Work out the finished part from the listing and answer in its coordinate system (mm). A direction names the side the tool comes from. Coordinates: 2 decimals unless noted, no trailing zeros. Write each loop counter-clockwise with the first axis right and the second up, starting at its lowest first coordinate (ties: lowest second). Pieces come first, ordered by that corner, then holes. Notation, with made-up numbers: (7.5, 42) - (27.5, 42) arc R29 cw to (27.5, 63) - close; hole circle Ø5 at (16, 87.5). An arc over 180 degrees is marked (long way). Use one line per item in the form item = value. Start each with the question number.
Item 1: Given pin 1 (2 mm diameter, centred on x = 1855, z = -24.5, fed in from +Y), flat-ended and moving along its own axis, determine where the tip first touches the part or whether it passes through.
Item 2: A cutting plane is placed at C-C (x = 1818). Write down the section's boundary in (y, z) (3 decimals).
Item 3: For faces 1 (the cylindrical face through (1867, -21, 28)), 2 (the flat face through (1773.643, -0.499, -36.897)), determine the directions among +Z, -Z, +X, -X, +Y, -Y from which every point of the face is accessible in a straight line to the end or side of a thin tool.
Item 4: A cutting plane is placed at B-B (y = 12). Write down the section's boundary in (x, z) (3 decimals).
Item 5: Consider probe 1 along X at (y, z) = (26.5, 31); probe 2 along X at (y, z) = (-8, -14); probe 3 along Y at (x, z) = (1794, -25.5) (1 decimal). Determine where each line is inside the solid, lowest interval first.
Item 6: A cutting plane is placed at A-A (z = 0). Write down the section's boundary in (x, y) (3 decimals).
Item 7: A cutting plane is placed at D-D (y = 29.5). Write down the section's boundary in (x, z) (3 decimals).
from build123d import *

# Parameters (mm, degrees)
SKETCH1_W           = 76.33
SKETCH1_H           = 76.33
BOSS_EXTRUDE1_DEPTH = 76.33
SKETCH2_R           = 35
BOSS_EXTRUDE2_DEPTH = 36.82
CHAMFER1_SIZE       = 2.5
CUT_EXTRUDE1_REACH  = 78.33
SKETCH3_R           = 18.71


with BuildPart() as part:
    # Sketch1 → Boss-Extrude1 (new body)
    with BuildSketch(Plane.ZY.offset(-1848.740517551)):
        Rectangle(SKETCH1_W, SKETCH1_H)
    extrude(amount=BOSS_EXTRUDE1_DEPTH)

    # Sketch2 → Boss-Extrude2 (add)
    with BuildSketch(Plane(origin=(1848.740517551, 0, 0), x_dir=(0, 0, -1), z_dir=(1, 0, 0))):
        Circle(SKETCH2_R)
    extrude(amount=BOSS_EXTRUDE2_DEPTH)

    # Chamfer1
    chamfer1_edges = [part.edges().sort_by_distance(p)[0] for p in [
        (1772.410517551, -38.165, 0),
        (1772.410517551, 0, -38.165),
        (1772.410517551, 38.165, 0),
        (1848.740517551, 0, -38.165),
        (1848.740517551, -38.165, 0),
        (1848.740517551, 0, 38.165),
        (1848.740517551, 38.165, 0),
        (1772.410517551, 0, 38.165),
        (1810.575517551, 38.165, -38.165),
        (1810.575517551, -38.165, -38.165),
        (1810.575517551, -38.165, 38.165),
        (1810.575517551, 38.165, 38.165),
    ]]
    chamfer(chamfer1_edges, length=CHAMFER1_SIZE)

    # Sketch3 → Cut-Extrude1 (cut, up to next)
    with BuildSketch(Plane(origin=(0, 0, -38.165), x_dir=(-1, 0, 0), z_dir=(0, 0, -1)), mode=Mode.PRIVATE) as cut_extrude1_sk1:
        with Locations((-1810.575517551, 0)):
            Circle(SKETCH3_R)
    cut_extrude1_tool1 = extrude(cut_extrude1_sk1.sketch, amount=-CUT_EXTRUDE1_REACH, mode=Mode.PRIVATE) & part.part
    add(cut_extrude1_tool1.solids().sort_by_distance((1810.575518, 0, -38.165))[0], mode=Mode.SUBTRACT)


solid = part.part
Answer:
q1.pin_1 = 25.94
q2.outline = (-38.165, -35.665) - (-35.665, -38.165) - (-17.174, -38.165) - (-17.174, 38.165) - (-35.665, 38.165) - (-38.165, 35.665) - close; (17.174, -38.165) - (35.665, -38.165) - (38.165, -35.665) - (38.165, 35.665) - (35.665, 38.165) - (17.174, 38.165) - close
q3.face_1 = +X
q3.face_2 = -Z, -X, +Y, -Y
q4.outline = (1772.411, -35.665) - (1774.911, -38.165) - (1796.221, -38.165) - (1796.221, 38.165) - (1774.911, 38.165) - (1772.411, 35.665) - close; (1824.93, -38.165) - (1846.241, -38.165) - (1848.741, -35.665) - (1848.741, -32.879) - (1885.561, -32.879) - (1885.561, 32.879) - (1848.741, 32.879) - (1848.741, 35.665) - (1846.241, 38.165) - (1824.93, 38.165) - close
q5.probe_1 = 1772.41 to 1848.74
q5.probe_2 = 1772.41 to 1793.66, 1827.49 to 1885.56
q5.probe_3 = -38.2 to -8.7, 8.7 to 38.2
q6.outline = (1772.411, -35.665) - (1774.911, -38.165) - (1846.241, -38.165) - (1848.741, -35.665) - (1848.741, -35) - (1885.561, -35) - (1885.561, 35) - (1848.741, 35) - (1848.741, 35.665) - (1846.241, 38.165) - (1774.911, 38.165) - (1772.411, 35.665) - close; hole circle Ø37.42 at (1810.576, 0)
q7.outline = (1772.411, -35.665) - (1774.911, -38.165) - (1846.241, -38.165) - (1848.741, -35.665) - (1848.741, -18.835) - (1885.561, -18.835) - (1885.561, 18.835) - (1848.741, 18.835) - (1848.741, 35.665) - (1846.241, 38.165) - (1774.911, 38.165) - (1772.411, 35.665) - close
